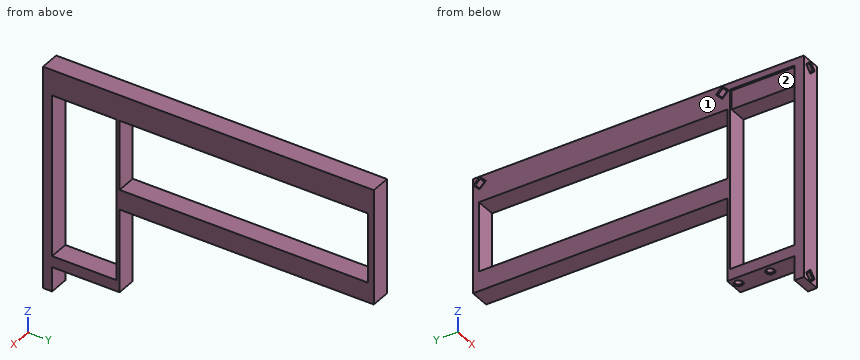
from build123d import *

# Parameters (mm, degrees)
SKETCH4_W                              = 44.704
SKETCH4_H                              = 159.004
SKETCH4_W_2                            = 103.7209
SKETCH4_H_2                            = 41.275
BOSS_EXTRUDE1_DEPTH                    = 12.7
F_18_0_1695_DIAMETER_HOLE1_D           = 4.3053
F_18_0_1695_DIAMETER_HOLE1_DEPTH       = 4.572
F_18_0_1695_DIAMETER_HOLE1_CSINK_D     = 5.5753
F_18_0_1695_DIAMETER_HOLE1_CSINK_ANGLE = 90
F_18_0_1695_DIAMETER_HOLE1_TIP         = 1.293442612
SKETCH11_W                             = 12.158133317
SKETCH11_H                             = 41.275
CUT_EXTRUDE3_DEPTH                     = 1.27
CUT_EXTRUDE1_DEPTH                     = 5.08
CUT_EXTRUDE2_DEPTH                     = 5.08
CHAMFER1_SIZE                          = 0.635


with BuildPart() as part:
    # Sketch4 → Boss-Extrude1 (new body)
    with BuildSketch(Plane(origin=(0, 0, 0), x_dir=(0, 0, -1), z_dir=(1, 0, 0))):
        Polygon((55.8038, 91.35), (-17.991666651, 91.35), (-17.991666651, -120.4686), (124.941666683, -120.4686), (124.941666683, -114.6186), (109.2327, -114.6186), (109.2327, -71.4386), (55.8038, -71.4386), align=None)
        with Locations((20.7518, 8.0634)):
            Rectangle(SKETCH4_W, SKETCH4_H, mode=Mode.SUBTRACT)
        with Locations((50.26025, -93.9811)):
            Rectangle(SKETCH4_W_2, SKETCH4_H_2, mode=Mode.SUBTRACT)
    extrude(amount=BOSS_EXTRUDE1_DEPTH)

    # #18 (0.1695) Diameter Hole1
    with Locations(Plane(origin=(0, 0, -109.2327), x_dir=(-1, 0, 0), z_dir=(0, 0, -1))):
        with Locations((-5.08, -95.6956), (-5.08, -75.3756)):
            CounterSinkHole(F_18_0_1695_DIAMETER_HOLE1_D / 2, F_18_0_1695_DIAMETER_HOLE1_CSINK_D / 2, depth=F_18_0_1695_DIAMETER_HOLE1_DEPTH, counter_sink_angle=F_18_0_1695_DIAMETER_HOLE1_CSINK_ANGLE)
            with Locations((0, 0, -(F_18_0_1695_DIAMETER_HOLE1_DEPTH + F_18_0_1695_DIAMETER_HOLE1_TIP / 2))):  # 118° drill point
                Cone(0, F_18_0_1695_DIAMETER_HOLE1_D / 2, F_18_0_1695_DIAMETER_HOLE1_TIP, mode=Mode.SUBTRACT)

    # Sketch11 → Cut-Extrude3 (cut)
    with BuildSketch(Plane.ZY):
        with Locations((7.679266659, -93.9811)):
            Rectangle(SKETCH11_W, SKETCH11_H)
    extrude(amount=-CUT_EXTRUDE3_DEPTH, mode=Mode.SUBTRACT)

    # Sketch9 → Cut-Extrude1 (cut)
    with BuildSketch(Plane.XZ.offset(120.4686)):
        Polygon((3.175, 13.758333317), (6.35, 16.933333317), (9.525, 13.758333317), (6.35, 10.583333317), align=None)
        Polygon((3.175, -120.708333349), (6.35, -117.533333349), (9.525, -120.708333349), (6.35, -123.883333349), align=None)
    extrude(amount=-CUT_EXTRUDE1_DEPTH, mode=Mode.SUBTRACT)

    # Sketch10 → Cut-Extrude2 (cut)
    with BuildSketch(Plane.ZY):
        Polygon((13.758333317, 90.291666667), (16.933333317, 87.116666667), (13.758333317, 83.941666667), (10.583333317, 87.116666667), align=None)
        Polygon((13.758333317, -65.0886), (16.933333317, -68.2636), (13.758333317, -71.4386), (10.583333317, -68.2636), align=None)
    extrude(amount=-CUT_EXTRUDE2_DEPTH, mode=Mode.SUBTRACT)

    # Chamfer1
    chamfer1_edges = [part.edges().sort_by_distance(p)[0] for p in [
        (5.08, 88.704166667, 12.170833317),
        (5.08, 88.704166667, 15.345833317),
        (5.08, 85.529166667, 15.345833317),
        (5.08, 85.529166667, 12.170833317),
        (0, 88.704166667, 12.170833317),
        (0, 85.529166667, 12.170833317),
        (0, 85.529166667, 15.345833317),
        (0, 88.704166667, 15.345833317),
        (5.08, -66.6761, 12.170833317),
        (5.08, -66.6761, 15.345833317),
        (5.08, -69.8511, 15.345833317),
        (5.08, -69.8511, 12.170833317),
        (0, -66.6761, 12.170833317),
        (0, -69.8511, 12.170833317),
        (0, -69.8511, 15.345833317),
        (0, -66.6761, 15.345833317),
        (4.7625, -115.3886, 12.170833317),
        (4.7625, -115.3886, 15.345833317),
        (7.9375, -115.3886, 15.345833317),
        (7.9375, -115.3886, 12.170833317),
        (4.7625, -120.4686, 12.170833317),
        (7.9375, -120.4686, 12.170833317),
        (7.9375, -120.4686, 15.345833317),
        (4.7625, -120.4686, 15.345833317),
        (4.7625, -115.3886, -122.295833349),
        (4.7625, -115.3886, -119.120833349),
        (7.9375, -115.3886, -119.120833349),
        (7.9375, -115.3886, -122.295833349),
        (4.7625, -120.4686, -122.295833349),
        (7.9375, -120.4686, -122.295833349),
        (7.9375, -120.4686, -119.120833349),
        (4.7625, -120.4686, -119.120833349),
    ]]
    chamfer(chamfer1_edges, length=CHAMFER1_SIZE)


solid = part.part
The model under review builds one solid part; all positions refer to its coordinate system, in mm. Face numbers are marked on the shaded views. Round coordinates to 2 decimals unless told otherwise and drop trailing zeros. Loops run counter-clockwise (first coordinate to the right, second up) from the corner with the lowest first, then second, coordinate; pieces in that order, holes last. Notation, with made-up numbers: M 17,48.5 L 24,48.5 A24 ccw 24,58.5 Z; hole C 37,75 d6. An arc over 180 degrees is marked long. Answer as a JSON object with one key per item and string values.
Item 1: We need section B-B, the plane z = -97.5. State the section outline as (x, y) points, and give its area (3 significant figures).
Check sheet entries:
{"outline": "M 0,-120.47 L 12.7,-120.47 L 12.7,-114.62 L 0,-114.62 Z; M 0,-73.34 L 12.7,-73.34 L 12.7,-71.44 L 0,-71.44 Z", "area": "98.5 mm2"}
Item 2: For line 1 along Y through (x, z) = (5.08, -107); line 2 along Y through (x, z) = (6.25, 1); line 3 along Z through (x, y) = (3.75, -55), list the stretches that pass through material, from the lowest coordinate up.
Check sheet entries:
{"line 1": "-120.47 to -97.85, -93.54 to -77.53, -73.22 to -71.44", "line 2": "-120.47 to -114.62, -73.34 to -71.44, 87.57 to 91.35", "line 3": "-55.8 to -43.1, 1.6 to 17.99"}
Item 3: We need section A-A, the plane y = -46.5. State the section outline as (x, z) points, and give its area (3 significant figures).
Check sheet entries:
{"outline": "M 0,-55.8 L 12.7,-55.8 L 12.7,-43.1 L 0,-43.1 Z; M 0,1.6 L 12.7,1.6 L 12.7,17.99 L 0,17.99 Z", "area": "369 mm2"}
Item 4: Clearance check with flat-ended pins moving along their axes: P1, Ø1.4, axis at y = 86.5, z = 14, coming from the -X side; P2, Ø6.5, axis at x = 8.5, z = -117, coming from the +Y side; P3, Ø6, axis at x = 11.5, y = -54, coming from the -Z side; P4, Ø8, axis at y = -37, z = -52.5, coming from the -X side. State where each tip first meets the part, or that it passes through.
Check sheet entries:
{"P1": "x = 5.08", "P2": "y = -114.62", "P3": "z = -55.8", "P4": "x = 0"}
Item 5: The part is to be moulded in two halves that separate along Z. For the marked faces 1 and 2, say which applies: +Z half, -Z half, draft (parallel to the pull), parting line (faces both ways), or undercut.
Check sheet entries:
{"face 1": "draft", "face 2": "undercut"}
